```python
from build123d import *

# Parameters (mm, degrees)
F0_R     = 9.525
F1_DEPTH = 25.4
F3_DEPTH = 25.401
F4_DEPTH = 11.0998
F6_DEPTH = 9.525


with BuildPart() as f1:
    # F0 (on Front) → F1 (new body)
    with BuildSketch(Plane.XZ):
        Circle(F0_R)
    extrude(amount=-F1_DEPTH)

    # F2 (on face) → F3 (cut, through all)
    with BuildSketch(Plane(origin=(0, 25.4, 0), x_dir=(-1, 0, 0), z_dir=(0, 1, 0))):
        with BuildLine():
            ThreePointArc((-4.7625, 0), (-3.367596, -3.367596), (0, -4.7625))
            ThreePointArc((0, -4.7625), (3.367596, -3.367596), (4.7625, 0))
            ThreePointArc((4.7625, 0), (3.367596, 3.367596), (0, 4.7625))
            ThreePointArc((0, 4.7625), (-3.367596, 3.367596), (-4.7625, 0))
        make_face()
    extrude(amount=-F3_DEPTH, mode=Mode.SUBTRACT)

    # F2 (on face) → F4 (cut)
    with BuildSketch(Plane(origin=(0, 25.4, 0), x_dir=(-1, 0, 0), z_dir=(0, 1, 0))):
        with BuildLine():
            Line((0, -4.7625), (4.7625, -4.7625))
            Line((4.7625, -4.7625), (4.7625, 0))
            ThreePointArc((4.7625, 0), (3.367596, -3.367596), (0, -4.7625))
        make_face()
        with BuildLine():
            Line((-4.7625, -4.7625), (0, -4.7625))
            ThreePointArc((0, -4.7625), (-3.367596, -3.367596), (-4.7625, 0))
            Line((-4.7625, 0), (-4.7625, -4.7625))
        make_face()
        with BuildLine():
            ThreePointArc((0, 4.7625), (3.367596, 3.367596), (4.7625, 0))
            Line((4.7625, 0), (4.7625, 4.7625))
            Line((4.7625, 4.7625), (0, 4.7625))
        make_face()
        with BuildLine():
            Line((-4.7625, 4.7625), (-4.7625, 0))
            ThreePointArc((-4.7625, 0), (-3.367596, 3.367596), (0, 4.7625))
            Line((0, 4.7625), (-4.7625, 4.7625))
        make_face()
    extrude(amount=-F4_DEPTH, mode=Mode.SUBTRACT)

    # F5 (on face) → F6 (cut)
    with BuildSketch(Plane.XZ):
        Polygon((3.704864, -6.293196), (7.3025, 0.061908), (3.597636, 6.355105), (-3.704864, 6.293196), (-7.3025, -0.061908), (-3.597636, -6.355105), align=None)
    extrude(amount=-F6_DEPTH, mode=Mode.SUBTRACT)


solid = f1.part
```
Verification items for the finished model (mm, model axes). A direction names the side the tool comes from. Coordinates: 2 decimals unless noted, no trailing zeros. Loops run counter-clockwise (first coordinate to the right, second up) from the corner with the lowest first, then second, coordinate; pieces in that order, holes last. Notation, with made-up numbers: (-33, 30.25) - (13, 30.25) arc R30 cw to (13, 66.25) - close; hole circle Ø2 at (-27.5, 28.25). An arc over 180 degrees is marked (long way). Return JSON: item names as keys, results as strings.
1. Thickness scan on L1, parallel to Z at x = 0, y = 10.25 (1 decimal); L2, parallel to Y at x = 6.25, z = -0.75 (3 decimals); L3, parallel to Z at x = -2.5, y = 21.25. Record the ranges inside material, lowest first.
Established:
{"L1": "z = -9.5 to -4.8, 4.8 to 9.5", "L2": "y = 9.525 to 25.4", "L3": "z = -9.19 to -4.76, 4.76 to 9.19"}
2. Tool access check on faces 4 (the flat face through (-5.48, 4.7, -3.16)), 5 (the flat face through (6.2, 0, 2.3)), 6 (the flat face through (4.762, 20, 0)). Record the directions out of +Z, -Z, +X, -X, +Y, -Y that give a thin tool (end or side, any length) a straight path to the whole face; none if there is none.
Established:
{"face 4": "-Y", "face 5": "+Z, -Z, +X, -X, -Y", "face 6": "+Y"}
3. Section check D-D, the plane x = 7. Record the boundary of the cut face in (y, z) (3 decimals).
Established:
{"outline": "(0, -6.46) - (25.4, -6.46) - (25.4, 6.46) - (0, 6.46) - (0, 0.576) - (9.525, 0.576) - (9.525, -0.472) - (0, -0.472) - close"}
4. Section check B-B, the plane x = 2.75. Record the boundary of the cut face in (y, z) (1 decimal), then the cut area to 3 significant figures.
Established:
{"outline": "(0, -9.1) - (25.4, -9.1) - (25.4, -4.8) - (14.3, -4.8) - (14.3, -3.9) - (9.5, -3.9) - (9.5, -6.3) - (0, -6.3) - close; (0, 6.3) - (9.5, 6.3) - (9.5, 3.9) - (14.3, 3.9) - (14.3, 4.8) - (25.4, 4.8) - (25.4, 9.1) - (0, 9.1) - close", "area": "200 mm2"}
5. Section check C-C, the plane z = -5.5. Record the boundary of the cut face in (x, y) (3 decimals), then the cut area to 3 significant figures.
Established:
{"outline": "(-7.777, 0) - (-4.101, 0) - (-4.101, 9.525) - (4.154, 9.525) - (4.154, 0) - (7.777, 0) - (7.777, 25.4) - (-7.777, 25.4) - close", "area": "316 mm2"}
6. Mould release check, pull along X, two halves, no side actions. Record for faces 1 (the flat face through (0, 25.4, -6)), 2 (the cylindrical face through (-7.559, 12.522, -5.796)), 3 (the flat face through (5.48, 4.7, 3.16)): +X half, -X half, draft (parallel to the pull), parting line (faces both ways), or undercut.
Established:
{"face 1": "draft", "face 2": "parting line", "face 3": "undercut"}
7. Go/stop test with flat-tipped pins: pin 1 (1.5 mm diameter, centred on x = -2.5, y = 11.5, fed in from -Z); pin 2 (4 mm diameter, centred on x = 3, z = 1.5, fed in from -Y) (3 decimals); pin 3 (4 mm diameter, centred on y = 21, z = -4.5, fed in from +X). Record where each tip stops, or that it passes through.
Established:
{"pin 1": "stops at z = -9.36", "pin 2": "stops at y = 9.525", "pin 3": "stops at x = 9.19"}
